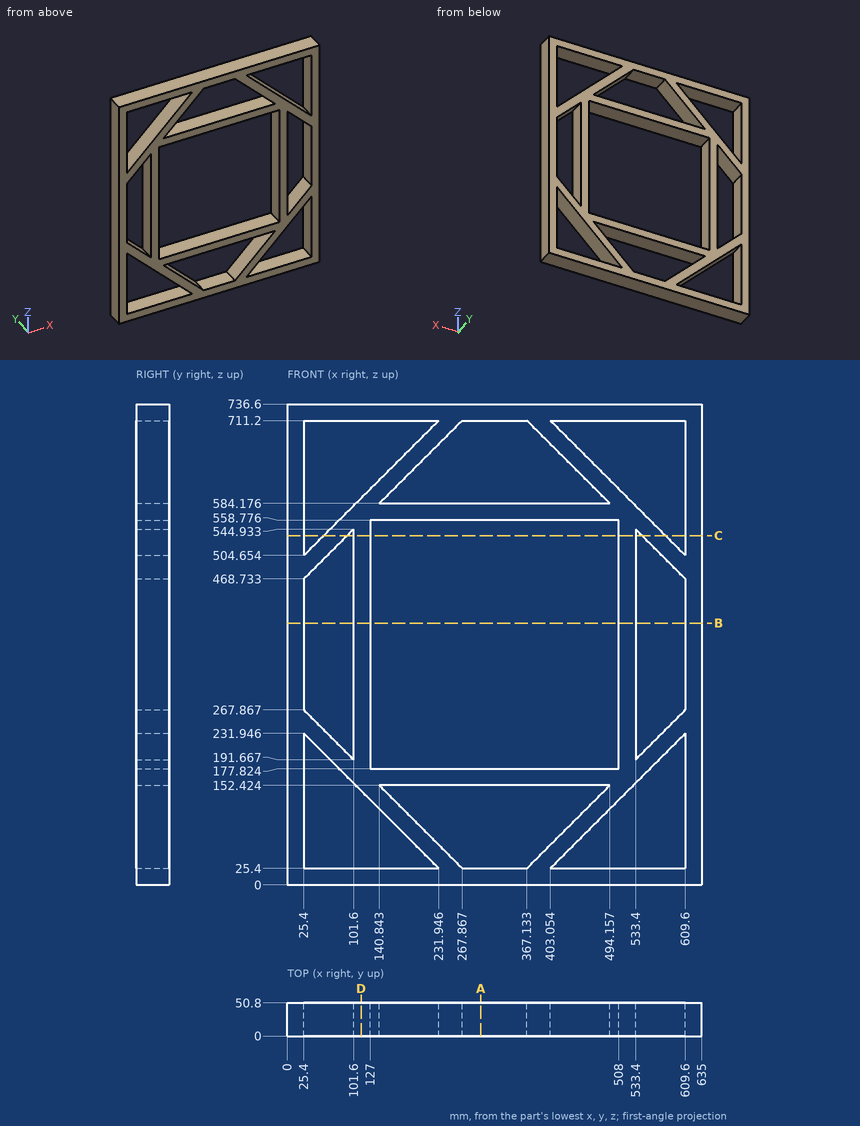
Geometry: see drawing. Coordinates: mm, zero at the bounding-box minimum. Give positions to 0.01 mm unless a question says otherwise; leave off trailing zeros. Order: outer loops, then holes, each group sorted by start corner. A loop starts at its lowest first (then second) coordinate and runs counter-clockwise, first axis right, second up.
Q1. Section B-B on z = 401. Output: boundary loops of the cut face in (x, y), and give its area (3 significant figures).
Checked values:
outline: (0, 0) - (25.4, 0) - (25.4, 50.8) - (0, 50.8) - close; (101.6, 0) - (127, 0) - (127, 50.8) - (101.6, 50.8) - close; (508, 0) - (533.4, 0) - (533.4, 50.8) - (508, 50.8) - close; (609.6, 0) - (635, 0) - (635, 50.8) - (609.6, 50.8) - close
area: 5,160 mm2
Q2. Section C-C on z = 535. Output: boundary loops of the cut face in (x, y), and give its area (3 significant figures).
Checked values:
outline: (0, 0) - (25.4, 0) - (25.4, 50.8) - (0, 50.8) - close; (55.75, 0) - (91.67, 0) - (91.67, 50.8) - (55.75, 50.8) - close; (101.6, 0) - (127, 0) - (127, 50.8) - (101.6, 50.8) - close; (508, 0) - (533.4, 0) - (533.4, 50.8) - (508, 50.8) - close; (543.33, 0) - (579.25, 0) - (579.25, 50.8) - (543.33, 50.8) - close; (609.6, 0) - (635, 0) - (635, 50.8) - (609.6, 50.8) - close
area: 8,810 mm2
Q3. Contact query for a flat-ended pin moving along its axis: pin 1 Ø15 at (y, z) = (38, 322) entering from -X. Output: stop coordinate, or through.
Checked values:
pin 1: stops at x = 0
Q4. Section D-D on x = 113. Output: boundary loops of the cut face in (y, z), and give its area (3 significant figures).
Checked values:
outline: (0, 0) - (50.8, 0) - (50.8, 25.4) - (0, 25.4) - close; (0, 144.35) - (50.8, 144.35) - (50.8, 592.25) - (0, 592.25) - close; (0, 711.2) - (50.8, 711.2) - (50.8, 736.6) - (0, 736.6) - close
area: 25,300 mm2
Q5. Section A-A on x = 296.5. Output: boundary loops of the cut face in (y, z), and give its area (3 significant figures).
Checked values:
outline: (0, 0) - (50.8, 0) - (50.8, 25.4) - (0, 25.4) - close; (0, 152.42) - (50.8, 152.42) - (50.8, 177.82) - (0, 177.82) - close; (0, 558.78) - (50.8, 558.78) - (50.8, 584.18) - (0, 584.18) - close; (0, 711.2) - (50.8, 711.2) - (50.8, 736.6) - (0, 736.6) - close
area: 5,160 mm2
Q6. Ray query, probe 1 along X at (y, z) = (29, 297.5); probe 2 along Z at (x, y) = (294.5, 26); probe 3 along X at (y, z) = (33.5, 66). Return the intervals inside material, ascending.
Checked values:
probe 1: x = 0 to 25.4, 101.6 to 127, 508 to 533.4, 609.6 to 635
probe 2: z = 0 to 25.4, 152.42 to 177.82, 558.78 to 584.18, 711.2 to 736.6
probe 3: x = 0 to 25.4, 191.35 to 227.27, 407.73 to 443.65, 609.6 to 635
